```python
from build123d import *

# Parameters (mm, degrees)
F0_W     = 250
F0_H     = 75
F1_DEPTH = 6.35
F2_W     = 25
F2_H     = 6.35
F3_DEPTH = 6.35
F4_W     = 220
F4_H     = 20
F5_DEPTH = 25
F6_W     = 6.35
F6_H     = 10
F6_H_2   = 12.5
F6_H_3   = 16.35
F7_DEPTH = 6.35


# Not quite as in the source:
# - a length typed as a fraction of an inch, garbled in the dataset ("3 / 203.2 mm" for 3/8 in), is restored


with BuildPart() as f1:
    # F0 (on Top) → F1 (new body)
    with BuildSketch(Plane.XY):
        Rectangle(F0_W, F0_H)
    extrude(amount=F1_DEPTH)

    # F2 (on face) → F3 (join, through all)
    with BuildSketch(Plane.XY.offset(6.35)):
        with Locations((-87.5, -40.675)):
            Rectangle(F2_W, F2_H)
        with Locations((-29.17, -40.675)):
            Rectangle(F2_W, F2_H)
        with Locations((29.16, -40.675)):
            Rectangle(F2_W, F2_H)
        with Locations((87.49, -40.675)):
            Rectangle(F2_W, F2_H)
    extrude(amount=-F3_DEPTH)

    # F4 (on face) → F5 (cut)
    with BuildSketch(Plane.XY.offset(6.35)):
        with Locations((0, -25.5)):
            Rectangle(F4_W, F4_H)
    extrude(amount=-F5_DEPTH, mode=Mode.SUBTRACT)

    # F6 (on face) → F7 (cut, through all)
    with BuildSketch(Plane.XY.offset(6.35)):
        with Locations((121.825, 32.5)):
            Rectangle(F6_W, F6_H)
        with Locations((121.825, 11.25)):
            Rectangle(F6_W, F6_H_2)
        with Locations((121.825, -11.25)):
            Rectangle(F6_W, F6_H_2)
        with Locations((121.825, -35.675)):
            Rectangle(F6_W, F6_H_3)
        with Locations((-121.825, -35.675)):
            Rectangle(F6_W, F6_H_3)
        with Locations((-121.825, 32.5)):
            Rectangle(F6_W, F6_H)
        with Locations((-121.825, 11.25)):
            Rectangle(F6_W, F6_H_2)
        with Locations((-121.825, -11.25)):
            Rectangle(F6_W, F6_H_2)
    extrude(amount=-F7_DEPTH, mode=Mode.SUBTRACT)


solid = f1.part
```
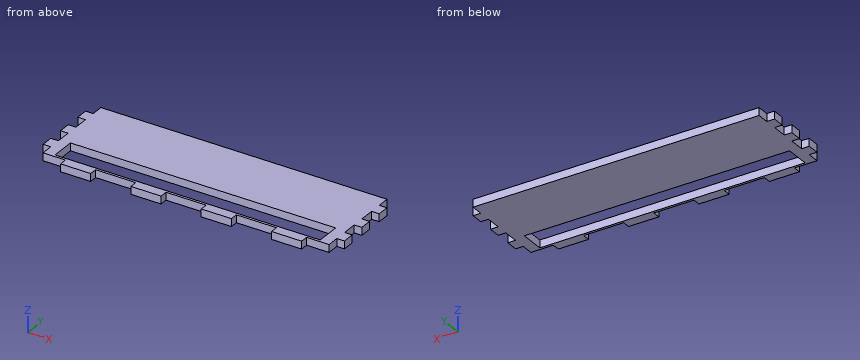
Geometry check sheet. Reference: the model listing, model coordinates, mm. Give positions to 0.01 mm unless a question says otherwise; leave off trailing zeros. Order: outer loops, then holes, each group sorted by start corner. A loop starts at its lowest first (then second) coordinate and runs counter-clockwise, first axis right, second up.
1. Gauge pin test, flat ends, axial feed: pin 1 Ø3 at (y, z) = (-11, 3) entering from -X; pin 2 Ø1.9 at (x, z) = (-108.5, 3) entering from -Y; pin 3 Ø10 at (x, y) = (8.5, 18) entering from -Z; pin 4 Ø3 at (x, z) = (-122.5, 4) entering from +Y. Record the tip position at first contact, or that the pin passes through.
2. Section check B-B, the plane y = 13. Enter the section's corners in (x, z), and give its area (3 significant figures).
3. Thickness scan on L1, parallel to Y at x = 104.5, z = 3.5; L2, parallel to Y at x = 34.5, z = 1.75; L3, parallel to X at y = -33.5, z = 0.75. Record the ranges inside material, lowest first.
4. Section check A-A, the plane x = 102.5. Enter the section's corners in (y, z).
Values follow:
1. pin 1: stops at x = -118.65
1. pin 2: stops at y = -37.5
1. pin 3: stops at z = 0
1. pin 4: stops at y = 27.5
2. outline: (-118.65, 0) - (118.65, 0) - (118.65, 6.35) - (-118.65, 6.35) - close
2. area: 1,510 mm2
3. L1: y = -37.5 to -35.5, -15.5 to 37.5
3. L2: y = -43.85 to -35.5, -15.5 to 37.5
3. L3: x = -118.65 to -110, 110 to 118.65
4. outline: (-37.5, 0) - (-35.5, 0) - (-35.5, 6.35) - (-37.5, 6.35) - close; (-15.5, 0) - (37.5, 0) - (37.5, 6.35) - (-15.5, 6.35) - close
